Geometry check sheet. Reference: drawing and pictorial views, mm from the part's lowest x, y, z. A direction names the side the tool comes from. Give positions to 0.01 mm unless a question says otherwise; leave off trailing zeros. Write each loop counter-clockwise with the first axis right and the second up, starting at its lowest first coordinate (ties: lowest second). Pieces come first, ordered by that corner, then holes. Notation, with made-up numbers: (8.5, -19) - (37.5, -19) arc R22 ccw to (37.5, 5) - close; hole circle Ø2 at (83, 33). An arc over 180 degrees is marked (long way). Put each result on its own line as item: value.
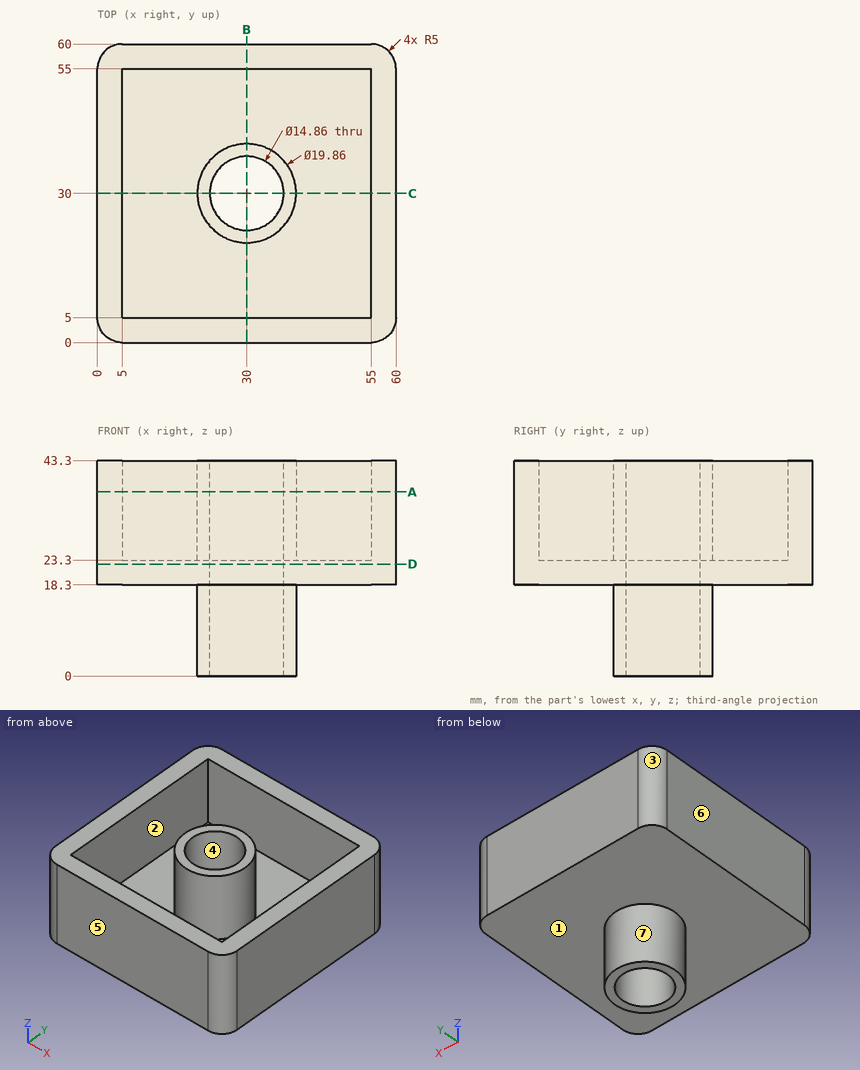
Q1. Release check for a two-part mould opening along X. For the marked faces 4, 5, 6 and 7 record: released by +X, released by -X, zero draft, split by the parting line, or undercut.
Answers follow:
face 4: undercut
face 5: zero draft
face 6: released by -X
face 7: split by the parting line
Q2. Set-up check for the marked faces 1, 2 and 3: record each of +Z, -Z, +X, -X, +Y, -Y from which the full face is reachable in a straight line by a thin tool's end or side.
Answers follow:
face 1: -Z
face 2: +Z
face 3: +Z, -Z, -X, +Y
Q3. Section check D-D, the plane z = 22.5. Record the cut outline in (x, y), plus the area to 3 significant figures.
Answers follow:
outline: (0, 5) arc R5 ccw to (5, 0) - (55, 0) arc R5 ccw to (60, 5) - (60, 55) arc R5 ccw to (55, 60) - (5, 60) arc R5 ccw to (0, 55) - close; hole circle Ø14.86 at (30, 30)
area: 3,410 mm2
Q4. Go/stop test with flat-tipped pins: pin 1 Ø3 at (x, z) = (26, 10.5) entering from +Y; pin 2 Ø10 at (y, z) = (16, 9) entering from -X; pin 3 Ø8 at (y, z) = (12.5, 11) entering from -X; pin 4 Ø5 at (x, y) = (28, 9) entering from -Z. Record where each tip stops, or that it passes through.
Answers follow:
pin 1: stops at y = 39.61
pin 2: stops at x = 25.8
pin 3: passes through
pin 4: stops at z = 18.3
Q5. Section check A-A, the plane z = 37. Record the cut outline in (x, y).
Answers follow:
outline: (0, 5) arc R5 ccw to (5, 0) - (55, 0) arc R5 ccw to (60, 5) - (60, 55) arc R5 ccw to (55, 60) - (5, 60) arc R5 ccw to (0, 55) - close; circle Ø19.86 at (30, 30); hole (5, 5) - (55, 5) - (55, 55) - (5, 55) - close; hole circle Ø14.86 at (30, 30)
Q6. Scan lines: line 1 along Y through (x, z) = (30, 29.5); line 2 along X through (y, z) = (29, 39); line 3 along Y through (x, z) = (30, 12). Record each from-to range of solid material in increasing order.
Answers follow:
line 1: y = 0 to 5, 20.07 to 22.57, 37.43 to 39.93, 55 to 60
line 2: x = 0 to 5, 20.12 to 22.64, 37.36 to 39.88, 55 to 60
line 3: y = 20.07 to 22.57, 37.43 to 39.93
Q7. Section check B-B, the plane x = 30. Record the cut outline in (y, z).
Answers follow:
outline: (0, 18.3) - (20.07, 18.3) - (20.07, 0) - (22.57, 0) - (22.57, 43.3) - (20.07, 43.3) - (20.07, 23.3) - (5, 23.3) - (5, 43.3) - (0, 43.3) - close; (37.43, 0) - (39.93, 0) - (39.93, 18.3) - (60, 18.3) - (60, 43.3) - (55, 43.3) - (55, 23.3) - (39.93, 23.3) - (39.93, 43.3) - (37.43, 43.3) - close
